For this review, take the finished solid that the model builds, in its own axes (mm). Coordinates: 2 decimals unless noted, no trailing zeros. Write each loop counter-clockwise with the first axis right and the second up, starting at its lowest first coordinate (ties: lowest second). Pieces come first, ordered by that corner, then holes.
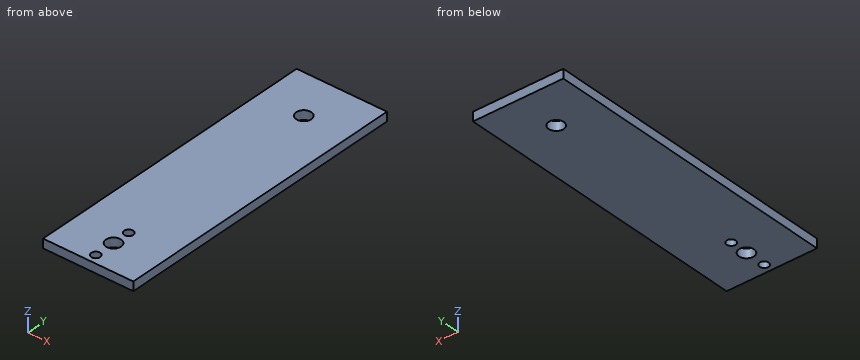
Autodesk Inventor part; units mm, degrees
ref_plane "YZ Plane" through (0, 0, 0) normal (1, 0, 0) x (0, 1, 0)
ref_plane "XZ Plane" through (0, 0, 0) normal (0, 1, 0) x (-1, 0, 0)
ref_plane "XY Plane" through (0, 0, 0) normal (0, 0, 1) x (1, 0, 0)
sketch "スケッチ1" plane through (0, 0, 0) normal (0, 0, 1) x (1, 0, 0)
  line L0 (0, 0) -> (30, 0)
  line L1 (30, 0) -> (30, 100)
  line L2 (30, 100) -> (0, 100)
  line L3 (0, 100) -> (0, 0)
  dimension "d0" = 100
  dimension "d1" = 30
extrude "押し出し1" add sketch "スケッチ1" along normal blind 3
sketch "スケッチ3" plane through (0, 0, 3) normal (0, 0, 1) x (1, 0, 0)
  circle A0 centre (15, 85) radius 2.5
  line L0 (30, 100) -> (0, 100)
  line L1 (0, 100) -> (0, 0)
  point P0 (15, 100)
  dimension "d9" = 5
  dimension "d10" = 15
  dimension "d11" = 15
extrude "押し出し3" cut sketch "スケッチ3" against normal blind 10
sketch "スケッチ4" plane through (0, 0, 3) normal (0, 0, 1) x (1, 0, 0)
  circle A0 centre (15, 10) radius 2.5
  line L0 (0, 0) -> (30, 0)
  line L1 (30, 0) -> (30, 100)
  dimension "d14" = 5
  dimension "d15" = 10
  dimension "d16" = 15
extrude "押し出し4" cut sketch "スケッチ4" against normal blind 10
sketch "スケッチ5" plane through (0, 0, 3) normal (0, 0, 1) x (1, 0, 0)
  circle A0 centre (15, 10) radius 2.5
  line L0 (15, 10) -> (15, 26.1579)
  line L1 (15, 26.1579) -> (15, -6.7471)
  line L2 (0, 0) -> (30, 0)
  point P0 (15, 16)
  point P1 (15, 3)
  dimension "d19" = 3
  dimension "d20" = 13
hole "穴1" at (15, 16, 3) at (15, 3, 3) direction (0, 0, -1) diameter 3 end through all
equation "\"d11\" = d10"
properties part number "practice_parts02"
1) Consider section A-A (x = 15). Give the boundary of the cut face in (y, z), then the cut area to 3 significant figures.
2) Consider section D-D (y = 84). Give the boundary of the cut face in (x, z), then the cut area to 3 significant figures.
3) Consider section C-C (z = 2.05). Give the boundary of the cut face in (x, y).
4) Consider section B-B (y = 16). Give the boundary of the cut face in (x, z), then the cut area to 3 significant figures.
5) For L1, parallel to Y at x = 15, z = 1.05; L2, parallel to Y at x = 16.75, z = 0.4; L3, parallel to X at y = 16, z = 1.8, list the stretches that pass through material, from the lowest coordinate up.
Results:
1. outline: (0, 0) - (1.5, 0) - (1.5, 3) - (0, 3) - close; (4.5, 0) - (7.5, 0) - (7.5, 3) - (4.5, 3) - close; (12.5, 0) - (14.5, 0) - (14.5, 3) - (12.5, 3) - close; (17.5, 0) - (82.5, 0) - (82.5, 3) - (17.5, 3) - close; (87.5, 0) - (100, 0) - (100, 3) - (87.5, 3) - close
1. area: 252 mm2
2. outline: (0, 0) - (12.71, 0) - (12.71, 3) - (0, 3) - close; (17.29, 0) - (30, 0) - (30, 3) - (17.29, 3) - close
2. area: 76.3 mm2
3. outline: (0, 0) - (30, 0) - (30, 100) - (0, 100) - close; hole circle Ø5 at (15, 10); hole circle Ø5 at (15, 85); hole circle Ø3 at (15, 3); hole circle Ø3 at (15, 16)
4. outline: (0, 0) - (13.5, 0) - (13.5, 3) - (0, 3) - close; (16.5, 0) - (30, 0) - (30, 3) - (16.5, 3) - close
4. area: 81.0 mm2
5. L1: y = 0 to 1.5, 4.5 to 7.5, 12.5 to 14.5, 17.5 to 82.5, 87.5 to 100
5. L2: y = 0 to 8.21, 11.79 to 83.21, 86.79 to 100
5. L3: x = 0 to 13.5, 16.5 to 30
